The listing builds one solid part. Answer for the finished solid, in the listing's coordinates (mm). A direction names the side the tool comes from. Give positions to 0.01 mm unless a question says otherwise; leave off trailing zeros. Order: outer loops, then holes, each group sorted by start corner. A loop starts at its lowest first (then second) coordinate and runs counter-clockwise, first axis right, second up. Notation, with made-up numbers: (-18.75, 8.5) - (24.25, 8.5) arc R12 cw to (24.25, 23.5) - close; hole circle Ø11 at (-28.5, 50). An arc over 180 degrees is marked (long way). Use CSV: the item, a comma, the result in double quotes.
Autodesk Inventor part; units mm, degrees
ref_plane "YZ Plane" through (0, 0, 0) normal (1, 0, 0) x (0, 1, 0)
ref_plane "XZ Plane" through (0, 0, 0) normal (0, 1, 0) x (-1, 0, 0)
ref_plane "XY Plane" through (0, 0, 0) normal (0, 0, 1) x (1, 0, 0)
sketch "Sketch1" plane through (0, 0, 0) normal (0, 0, 1) x (1, 0, 0)
  line L0 (-20.6375, 7.9375) -> (20.6375, 7.9375)
  line L1 (20.6375, 7.9375) -> (20.6375, -7.9375)
  line L2 (20.6375, -7.9375) -> (-20.6375, -7.9375)
  line L3 (-20.6375, -7.9375) -> (-20.6375, 7.9375)
  point P0 (0, 0)
  point P1 (0, 7.9375)
  point P2 (-20.6375, 0)
  dimension "d0" = 41.275
  dimension "d1" = 15.875
extrude "Plate1" add sketch "Sketch1" along normal blind 1.524
sketch "Sketch3" plane through (-21.3995, -7.9375, 2.286) normal (-1, 0, 0) x (0, -1, 0)
  line L0 (-15.875, 0) -> (0, 0)
  line L1 (0, 0) -> (0, 0.254)
  line L2 (0, 0.254) -> (-15.875, 0.254)
  line L3 (-15.875, 0.254) -> (-15.875, 0)
edge flange "Flange1" height 2.54 angle 90 thickness 1.524 bend radius 0.762 thickness toward (-1, 0, 0) relief tear relief width 1.524 relief depth 0.762 edges at (-20.6375, 0, 1.524) wall of the first edge with corners at (-21.3995, 7.9375, 2.286) (-21.3995, -7.9375, 2.286) (-21.3995, -7.9375, 2.54) (-21.3995, 7.9375, 2.54)
bend "Bend1"
corner "Corner1"
sketch "Sketch4" plane through (21.3995, 7.9375, 2.286) normal (1, 0, 0) x (0, 1, 0)
  line L0 (-15.875, 0) -> (0, 0)
  line L1 (0, 0) -> (0, 0.254)
  line L2 (0, 0.254) -> (-15.875, 0.254)
  line L3 (-15.875, 0.254) -> (-15.875, 0)
edge flange "Flange2" height 2.54 angle 90 thickness 1.524 bend radius 0.762 thickness toward (1, 0, 0) relief tear relief width 1.524 relief depth 0.762 edges at (20.6375, 0, 1.524) wall of the first edge with corners at (21.3995, -7.9375, 2.286) (21.3995, 7.9375, 2.286) (21.3995, 7.9375, 2.54) (21.3995, -7.9375, 2.54)
bend "Bend2"
corner "Corner2"
sketch "Sketch7" plane through (-23.6855, 7.9375, 3.302) normal (0, 0, 1) x (1, 0, 0)
  line L0 (0, -15.875) -> (0, 0)
  line L1 (0, 0) -> (-21.5265, 0)
  line L2 (-21.5265, 0) -> (-21.5265, -15.875)
  line L3 (-21.5265, -15.875) -> (0, -15.875)
edge flange "Flange5" height 23.8125 angle 90 thickness 1.524 bend radius 0.762 thickness toward (0, 0, 1) relief tear relief width 1.524 relief depth 0.762 edges at (-22.9235, 0, 2.54) wall of the first edge with corners at (-23.6855, -7.9375, 3.302) (-23.6855, 7.9375, 3.302) (-45.212, 7.9375, 3.302) (-45.212, -7.9375, 3.302)
bend "Bend5"
corner "Corner5"
sketch "Sketch8" plane through (23.6855, -7.9375, 3.302) normal (0, 0, 1) x (1, 0, 0)
  line L0 (0, 15.875) -> (0, 0)
  line L1 (0, 0) -> (21.5265, 0)
  line L2 (21.5265, 0) -> (21.5265, 15.875)
  line L3 (21.5265, 15.875) -> (0, 15.875)
edge flange "Flange6" height 23.8125 angle 90 thickness 1.524 bend radius 0.762 thickness toward (0, 0, 1) relief tear relief width 1.524 relief depth 0.762 edges at (21.3995, 0, 2.54) wall of the first edge with corners at (23.6855, 7.9375, 3.302) (23.6855, -7.9375, 3.302) (45.212, -7.9375, 3.302) (45.212, 7.9375, 3.302)
bend "Bend6"
corner "Corner6"
sketch "Sketch9" plane through (-45.212, -7.9375, 3.302) normal (0, 0, -1) x (-1, 0, 0)
  line L0 (0, 0) -> (0, 15.875)
  point P0 (-45.212, 7.9375)
  point P1 (-7.112, 7.9375)
  point P2 (-83.312, 7.9375)
  point P3 (0, 7.9375)
  dimension "d65" = 76.2
  dimension "d66" = 7.112
hole "Hole1" at (-38.1, 0, 3.302) at (38.1, 0, 3.302) direction (0, 0, 1) diameter 3.302 depth 1.524 tip angle 118
fillet "Corner Round1" radius 3.175 4 edges at (-45.212, -7.9375, 4.064) (-45.212, 7.9375, 4.064) (45.212, 7.9375, 4.064) (45.212, -7.9375, 4.064)
equation "\"d72\" = Thickness"
equation "\"d2\" = Thickness"
equation "\"d5\" = BendReliefWidth"
equation "\"d6\" = BendReliefDepth"
equation "\"d7\" = MinimumRemnant"
equation "\"d8\" = TransitionRadius"
equation "\"d12\" = CornerReliefSize"
equation "\"d13\" = GapSize"
equation "\"d14\" = JacobiRadiusSize"
equation "\"d15\" = BendReliefWidth"
equation "\"d16\" = BendReliefDepth"
equation "\"d17\" = MinimumRemnant"
equation "\"d18\" = TransitionRadius"
equation "\"d22\" = CornerReliefSize"
equation "\"d23\" = GapSize"
equation "\"d24\" = JacobiRadiusSize"
equation "\"d45\" = BendReliefWidth"
equation "\"d46\" = BendReliefDepth"
equation "\"d47\" = MinimumRemnant"
equation "\"d48\" = TransitionRadius"
equation "\"d52\" = CornerReliefSize"
equation "\"d53\" = GapSize"
equation "\"d54\" = JacobiRadiusSize"
equation "\"d55\" = BendReliefWidth"
equation "\"d56\" = BendReliefDepth"
equation "\"d57\" = MinimumRemnant"
equation "\"d58\" = TransitionRadius"
equation "\"d62\" = CornerReliefSize"
equation "\"d63\" = GapSize"
equation "\"d64\" = JacobiRadiusSize"
equation "\"BendRadius\" = Thickness"
equation "\"BendReliefWidth\" = Thickness"
equation "\"BendReliefDepth\" = 0.5 * Thickness"
equation "\"CornerReliefSize\" = 4 * Thickness"
equation "\"MinimumRemnant\" = 2 * Thickness"
equation "\"TransitionRadius\" = BendRadius"
equation "\"JacobiRadiusSize\" = BendRadius"
equation "\"GapSize\" = Thickness"
properties part number "J010308" material "STAINLESS STEEL, 316"
Item 1: Each of these flat-tipped pins is pushed along its axis until it touches: pin 1 (8 mm diameter, centred on x = 34, y = -2, fed in from -Z); pin 2 (1.5 mm diameter, centred on x = -18, y = 1.5, fed in from +Z). Where does it stop, or does it pass through?
Taken from the geometry:
pin 1,"z = 3.3"
pin 2,"z = 1.52"
Item 2: Which of the six approach directions +Z, -Z, +X, -X, +Y, -Y give full straight-line access (tool end or side, diameter ignored) to faces 1 (the face through (-36.5, -0.4, 4.1)), 2 (the face through (34, 0, 3.302)), 3 (the face through (-34, 0, 3.302)), 4 (the face through (0, 0, 1.524)), 5 (the face through (-45.212, 0, 4))?
Taken from the geometry:
face 1,"+Z, -Z"
face 2,"-Z, +X, +Y, -Y"
face 3,"-Z, -X, +Y, -Y"
face 4,"+Z, +Y, -Y"
face 5,"+Z, -Z, -X, +Y, -Y"
Item 3: The part is cut by section B-B (y = 0). Give the vertices of the cut face in (x, z).
Taken from the geometry:
outline,"(-45.21, 3.3) - (-39.75, 3.3) - (-39.75, 4.83) - (-45.21, 4.83) - close; (-36.45, 3.3) - (-23.69, 3.3) arc R0.76 cw to (-22.92, 2.54) - (-22.92, 2.29) arc R2.29 ccw to (-20.64, 0) - (20.64, 0) arc R2.29 ccw to (22.92, 2.29) - (22.92, 2.54) arc R0.76 cw to (23.69, 3.3) - (36.45, 3.3) - (36.45, 4.83) - (23.69, 4.83) arc R2.29 ccw to (21.4, 2.54) - (21.4, 2.29) arc R0.76 cw to (20.64, 1.52) - (-20.64, 1.52) arc R0.76 cw to (-21.4, 2.29) - (-21.4, 2.54) arc R2.29 ccw to (-23.69, 4.83) - (-36.45, 4.83) - close; (39.75, 3.3) - (45.21, 3.3) - (45.21, 4.83) - (39.75, 4.83) - close"
Item 4: The part is cut by section C-C (y = -3.5). Give the vertices of the cut face in (x, z), and give its area (3 significant figures).
Taken from the geometry:
outline,"(-45.21, 3.3) - (-23.69, 3.3) arc R0.76 cw to (-22.92, 2.54) - (-22.92, 2.29) arc R2.29 ccw to (-20.64, 0) - (20.64, 0) arc R2.29 ccw to (22.92, 2.29) - (22.92, 2.54) arc R0.76 cw to (23.69, 3.3) - (45.21, 3.3) - (45.21, 4.83) - (23.69, 4.83) arc R2.29 ccw to (21.4, 2.54) - (21.4, 2.29) arc R0.76 cw to (20.64, 1.52) - (-20.64, 1.52) arc R0.76 cw to (-21.4, 2.29) - (-21.4, 2.54) arc R2.29 ccw to (-23.69, 4.83) - (-45.21, 4.83) - close"
area,"144 mm^2"
Item 5: Find the intervals of material crossed by line 1 along Y through (x, z) = (-38.1, 4.1); line 2 along X through (y, z) = (-0.25, 4.6); line 3 along Z through (x, y) = (27, 0), in increasing order.
Taken from the geometry:
line 1,"-7.94 to -1.65, 1.65 to 7.94"
line 2,"-45.21 to -39.73, -36.47 to -22.69, 22.69 to 36.47, 39.73 to 45.21"
line 3,"3.3 to 4.83"
Item 6: The part is cut by section A-A (x = 38.1). Give the vertices of the cut face in (y, z), and give its area (3 significant figures).
Taken from the geometry:
outline,"(-7.94, 3.3) - (-1.65, 3.3) - (-1.65, 4.83) - (-7.94, 4.83) - close; (1.65, 3.3) - (7.94, 3.3) - (7.94, 4.83) - (1.65, 4.83) - close"
area,"19.2 mm^2"
Item 7: The part is cut by section D-D (x = 17). Give the vertices of the cut face in (y, z).
Taken from the geometry:
outline,"(-7.94, 0) - (7.94, 0) - (7.94, 1.52) - (-7.94, 1.52) - close"
Item 8: The mould has two halves that part along X. Classify faces 6 (the face through (-22.087, 0.111, 4.174)), 7 (the face through (44.31, 6.98, 4.07)), 8 (the face through (-35, 0, 4.826)), 9 (the face through (-22.272, -0.111, 0.687)): +X half, -X half, draft (parallel to the pull), parting line (faces both ways), or undercut.
Taken from the geometry:
face 6,"undercut"
face 7,"+X half"
face 8,"draft"
face 9,"-X half"
